from build123d import *

# Parameters (mm, degrees)
SKETCH_1_W      = 6
SKETCH_1_H      = 10
SKETCH_1_W_2    = 112.5
SKETCH_1_H_2    = 20
EXTRUDE_1_DEPTH = 3
FILLET_1_R      = 0.5


with BuildPart() as part:
    # Эскиз1 → Бобышка-Вытянуть1 (new body)
    with BuildSketch(Plane(origin=(0, 0, 0), x_dir=(1, 0, 0), z_dir=(0, 1, 0))):
        with Locations((-59.25, 0)):
            Rectangle(SKETCH_1_W, SKETCH_1_H)
        Rectangle(SKETCH_1_W_2, SKETCH_1_H_2)
        with Locations((59.25, 0)):
            Rectangle(SKETCH_1_W, SKETCH_1_H)
    extrude(amount=EXTRUDE_1_DEPTH)

    # Скругление1
    fillet_1_edges = [part.edges().sort_by_distance(p)[0] for p in [
        (-62.25, 1.5, 5),
        (-62.25, 1.5, -5),
        (62.25, 1.5, -5),
        (62.25, 1.5, 5),
    ]]
    fillet(fillet_1_edges, radius=FILLET_1_R)


solid = part.part
For this review, take the finished solid that the model builds, in its own axes (mm). A direction names the side the tool comes from. Round coordinates to 2 decimals unless told otherwise and drop trailing zeros. Loops run counter-clockwise (first coordinate to the right, second up) from the corner with the lowest first, then second, coordinate; pieces in that order, holes last. Notation, with made-up numbers: (44.5, 77) - (57.5, 77) arc R6 ccw to (57.5, 86) - close; hole circle Ø7 at (49.25, -12.75). An arc over 180 degrees is marked (long way). One line per item, written item: value. Start each with the question number.
Item 1: For faces 1 (the flat face through (-59, 1, -5)), 2 (the flat face through (59, 1, -5)), 3 (the flat face through (-56.25, 1, 8)), list the 3-axis set-ups (+Z, -Z, +X, -X, +Y, -Y) from which the entire face can be reached by the end or side of a thin tool; tool diameter is ignored.
Item 2: Take a section at A-A (y = 0.9). Give the boundary of the cut face in (x, z).
Item 3: For L1, parallel to Z at x = 57, y = 0.5; L2, parallel to X at y = 1.6, z = 6.25, list the stretches that pass through material, from the lowest coordinate up.
Item 4: Clearance check with flat-ended pins moving along their axes: pin 1 Ø0.9 at (y, z) = (2, 7.5) entering from +X; pin 2 Ø1.5 at (x, y) = (58.5, 1) entering from +Z; pin 3 Ø1.5 at (y, z) = (2, 7.5) entering from -X. State where each tip first meets the part, or that it passes through.
Item 5: Take a section at B-B (z = 8.5). Give the boundary of the cut face in (x, y), plus the area to 4 significant figures.
Answer below:
1. face 1: -Z, -X, +Y, -Y
1. face 2: -Z, +X, +Y, -Y
1. face 3: +Z, -X, +Y, -Y
2. outline: (-62.25, -4.5) arc R0.5 ccw to (-61.75, -5) - (-56.25, -5) - (-56.25, -10) - (56.25, -10) - (56.25, -5) - (61.75, -5) arc R0.5 ccw to (62.25, -4.5) - (62.25, 4.5) arc R0.5 ccw to (61.75, 5) - (56.25, 5) - (56.25, 10) - (-56.25, 10) - (-56.25, 5) - (-61.75, 5) arc R0.5 ccw to (-62.25, 4.5) - close
3. L1: z = -5 to 5
3. L2: x = -56.25 to 56.25
4. pin 1: stops at x = 56.25
4. pin 2: stops at z = 5
4. pin 3: stops at x = -56.25
5. outline: (-56.25, 0) - (56.25, 0) - (56.25, 3) - (-56.25, 3) - close
5. area: 337.5 mm2
